from build123d import *

# Parameters (mm, degrees)
SKETCH1_R           = 15.5
BOSS_EXTRUDE1_DEPTH = 0.396875
SKETCH2_R           = 15.5
BOSS_EXTRUDE2_DEPTH = 0.396875
BOSS_EXTRUDE2_TAPER = 85
SKETCH3_R           = 3.75
BOSS_EXTRUDE3_DEPTH = 3
FILLET1_R           = 0.75
CUT_EXTRUDE1_DEPTH  = 0.79375
SKETCH5_R           = 2.5
CUT_EXTRUDE2_DEPTH  = 3


with BuildPart() as part:
    # Sketch1 → Boss-Extrude1 (new body)
    with BuildSketch(Plane.XY):
        Circle(SKETCH1_R)
    extrude(amount=BOSS_EXTRUDE1_DEPTH)

    # Sketch2 → Boss-Extrude2 (add)
    with BuildSketch(Plane.XY.offset(0.396875)):
        Circle(SKETCH2_R)
    extrude(amount=BOSS_EXTRUDE2_DEPTH, taper=BOSS_EXTRUDE2_TAPER)

    # Sketch3 → Boss-Extrude3 (add)
    with BuildSketch(Plane.XY.offset(0.79375)):
        Circle(SKETCH3_R)
    extrude(amount=BOSS_EXTRUDE3_DEPTH)

    # Fillet1
    fillet1_edges = [part.edges().sort_by_distance(p)[0] for p in [
        (-3.75, 0, 0.79375),
    ]]
    fillet(fillet1_edges, radius=FILLET1_R)

    # Sketch4 → Cut-Extrude1 (cut)
    with BuildSketch(Plane(origin=(0, 0, 0), x_dir=(-1, 0, 0), z_dir=(0, 0, -1))):
        with BuildLine():
            Line((-1.75, 1.75), (1.75, 1.75))
            ThreePointArc((1.75, 1.75), (3.5, 0), (1.75, -1.75))
            Line((1.75, -1.75), (-1.75, -1.75))
            ThreePointArc((-1.75, -1.75), (-3.5, 0), (-1.75, 1.75))
        make_face()
    extrude(amount=-CUT_EXTRUDE1_DEPTH, mode=Mode.SUBTRACT)

    # Sketch5 → Cut-Extrude2 (cut)
    with BuildSketch(Plane.XY.offset(3.79375)):
        Circle(SKETCH5_R)
    extrude(amount=-CUT_EXTRUDE2_DEPTH, mode=Mode.SUBTRACT)


solid = part.part
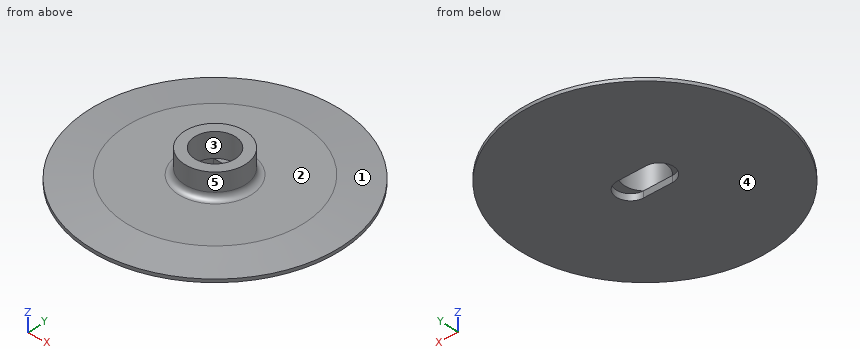
CAD build for the part. Positions are in the model's coordinates, mm. Face numbers are marked on the shaded views. A direction names the side the tool comes from. Round coordinates to 2 decimals unless told otherwise and drop trailing zeros. Order: outer loops, then holes, each group sorted by start corner. A loop starts at its lowest first (then second) coordinate and runs counter-clockwise, first axis right, second up. Notation, with made-up numbers: M 15,-2 L 45,-2 A19 cw 45,7 Z; hole C -23.5,70 d4. An arc over 180 degrees is marked long. Use one line per item in the form item = value.
Q1. Saw through at C-C on z = 2.4. Give the cut face in (x, y), then the cut area to 3 significant figures.
Recorded:
outline = C 0,0 d7.5; hole C 0,0 d5
area = 24.5 mm^2
Q2. Saw through at A-A on x = 0. Give the cut face in (y, z), then the cut area to 3 significant figures.
Recorded:
outline = M -15.5,0 L -1.75,0 L -1.75,0.79 L -2.5,0.79 L -2.5,3.79 L -3.75,3.79 L -3.75,1.54 A0.75 cw -4.5,0.79 L -10.96,0.79 L -15.5,0.4 Z; M 1.75,0 L 15.5,0 L 15.5,0.4 L 10.96,0.79 L 4.5,0.79 A0.75 cw 3.75,1.54 L 3.75,3.79 L 2.5,3.79 L 2.5,0.79 L 1.75,0.79 Z
area = 27.8 mm^2
Q3. Which spindle directions (+Z, -Z, +X, -X, +Y, -Y) get a long thin tool onto all of the face, cutting with end or side? Do the marked faces 4 and 5. Say none if no direction does.
Recorded:
face_4 = -Z, +X, -X, +Y, -Y
face_5 = +Z
Q4. Flat gauge pins, fed straight in: P1, Ø0.9, axis at x = -2.5, y = 0.5, coming from the -Z side; P2, Ø5, axis at x = -10.5, y = -11.5, coming from the +Z side. Where does each tip first touch, or does it go through?
Recorded:
P1 = 0.79
P2 = 0.61
Q5. Saw through at B-B on y = 0. Give the cut face in (x, z).
Recorded:
outline = M -15.5,0 L -3.5,0 L -3.5,0.79 L -2.5,0.79 L -2.5,3.79 L -3.75,3.79 L -3.75,1.54 A0.75 cw -4.5,0.79 L -10.96,0.79 L -15.5,0.4 Z; M 2.5,0.79 L 3.5,0.79 L 3.5,0 L 15.5,0 L 15.5,0.4 L 10.96,0.79 L 4.5,0.79 A0.75 cw 3.75,1.54 L 3.75,3.79 L 2.5,3.79 Z
Q6. Probe L1, parallel to Y at x = 0, z = 2.3; L2, parallel to Z at x = -6, y = -4.5; L3, parallel to X at y = 0.5, z = 2.25. List the from-to ranges inside material, lowest first.
Recorded:
L1 = -3.75 to -2.5, 2.5 to 3.75
L2 = 0 to 0.79
L3 = -3.72 to -2.45, 2.45 to 3.72
Q7. Two-plate mould, pull along Y, no slides. Class the marked faces 1, 2 and 3: +Y half, -Y half, draft (parallel to the pull), parting line (faces both ways), or undercut.
Recorded:
face_1 = parting line
face_2 = draft
face_3 = undercut
